For this review, take the finished solid that the model builds, in its own axes (mm). A direction names the side the tool comes from. Round coordinates to 2 decimals unless told otherwise and drop trailing zeros. Order: outer loops, then holes, each group sorted by start corner. A loop starts at its lowest first (then second) coordinate and runs counter-clockwise, first axis right, second up. Notation, with made-up numbers: (41.5, 81.25) -> (71.5, 81.25) arc R24 ccw to (71.5, 101.25) -> close; hole circle Ø9 at (-36, 10). An arc over 180 degrees is marked (long way). Use a Markdown table: item, result. Add a question column.
1) Wall thickness on line 1 along Y through (x, z) = (-21, 17); line 2 along X through (y, z) = (-2, 20.25); line 3 along Y through (x, z) = (-56, 3.5): over which ranges is each line inside the solid? List them lowest first. Write a range as [from, to].
2) Clearance check with flat-ended pins moving along their axes: P1, Ø2, axis at x = -53.6, z = 9.38, coming from the +Y side; P2, Ø5, axis at y = -20.5, z = 8.5, coming from the -X side; P3, Ø3, axis at y = -3.5, z = 14, coming from the +X side; P4, Ø4, axis at x = -54, z = 10.5, coming from the -Y side. State where each tip first meets the part, or that it passes through.
3) Machinability: for faces 4 (the face through (-10.201, -4, 18)), 5 (the face through (-55.077, -7.64, 8.434)), 6 (the face through (-54, -6.119, 14)), 7 (the face through (-28.201, -4, 15)), 8 (the face through (-54, -9.119, 14)), which of the approach directions +Z, -Z, +X, -X, +Y, -Y give a long, thin tool a straight path to every point of the face, cutting with its end or side? Answer none if there is none.
4) Consider section A-A (z = 19.5). State the section outline as (x, y) points, plus the area to 3 significant figures.
5) Consider section C-C (y = 2). State the section outline as (x, z) points, plus the area to 3 significant figures.
6) Draft analysis for pull direction Y (two halves, no side actions). For faces 1 (the face through (-21.87, -4.46, 5.98)), 2 (the face through (-50.401, 6, 14)), 3 (the face through (-31, 17.781, 14)), state which applies: pulls with the +Y half, pulls with the -Y half, needs draft (parallel to the pull), parting line crosses it, or undercut.
7) Consider section D-D (z = 5). State the section outline as (x, y) points.
8) Consider section B-B (x = -40.5). State the section outline as (y, z) points, plus the area to 3 significant figures.
```python
from build123d import *

# Parameters (mm, degrees)
SKETCH2_W               = 40.2
SKETCH2_H               = 43.15
BOSS_EXTRUDE1_DEPTH     = 29.13
SKETCH3_W               = 29.13
SKETCH3_H               = 3
BOSS_EXTRUDE2_DEPTH     = 8
CUT_EXTRUDE1_DEPTH      = 8
CUT_EXTRUDE1_DEPTH_BACK = 8
SKETCH4_R               = 1.75
SKETCH5_R               = 1.75
CUT_EXTRUDE2_DEPTH      = 40
SKETCH6_R               = 3
CUT_EXTRUDE3_DEPTH      = 18


with BuildPart() as part:
    # Sketch2 → Boss-Extrude1 (new body)
    with BuildSketch(Plane.XY):
        with Locations((-30.301325873, -3.793821583)):
            Rectangle(SKETCH2_W, SKETCH2_H)
    extrude(amount=BOSS_EXTRUDE1_DEPTH)

    # Sketch3 → Boss-Extrude2 (add)
    with BuildSketch(Plane.ZY.offset(50.401325873)):
        with Locations((14.565, -7.618821583)):
            Rectangle(SKETCH3_W, SKETCH3_H)
    extrude(amount=BOSS_EXTRUDE2_DEPTH)

    # Sketch4 → Cut-Extrude1 (cut, two sides: drawn at the far end of the back side and taken through both)
    with BuildSketch(Plane(origin=(0, -9.118821583, 0), x_dir=(1, 0, 0), z_dir=(0, 1, 0)).offset(-CUT_EXTRUDE1_DEPTH_BACK)):
        with Locations(Location((-53.601325886, -9.375, 0), (0, 0, 90))):
            Circle(SKETCH4_R)
        with Locations(Location((-53.601325886, -19.725, 0), (0, 0, 90))):
            Circle(SKETCH4_R)
    extrude(amount=CUT_EXTRUDE1_DEPTH + CUT_EXTRUDE1_DEPTH_BACK, mode=Mode.SUBTRACT)

    # Sketch5 → Cut-Extrude2 (cut)
    with BuildSketch(Plane(origin=(0, 0, 0), x_dir=(-1, 0, 0), z_dir=(0, 0, -1))):
        with Locations((40.351325873, -3.793821583)):
            Circle(SKETCH5_R)
        with Locations((20.251325873, -3.793821583)):
            Circle(SKETCH5_R)
    extrude(amount=-CUT_EXTRUDE2_DEPTH, mode=Mode.SUBTRACT)

    # Sketch6 → Cut-Extrude3 (cut)
    with BuildSketch(Plane(origin=(-10.201325873, 0, 0), x_dir=(0, 0, -1), z_dir=(1, 0, 0))):
        with Locations((-14.565, -3.793821583)):
            Circle(SKETCH6_R)
    extrude(amount=-CUT_EXTRUDE3_DEPTH, mode=Mode.SUBTRACT)


solid = part.part
```
Results list:
| question | item | result |
|---|---|---|
| 1 | line 1 | [-25.37, -5.55], [-2.04, 17.78] |
| 1 | line 2 | [-50.4, -10.2] |
| 1 | line 3 | [-9.12, -6.12] |
| 2 | P1 | through |
| 2 | P2 | x = -50.4 |
| 2 | P3 | x = -28.2 |
| 2 | P4 | y = -9.12 |
| 3 | face 4 | +Z, -Z, +X, +Y, -Y |
| 3 | face 5 | +Y, -Y |
| 3 | face 6 | +Z, -Z, -X, +Y |
| 3 | face 7 | +X |
| 3 | face 8 | +Z, -Z, -X, -Y |
| 4 | outline | (-58.4, -9.12) -> (-55.34, -9.12) -> (-55.34, -6.12) -> (-58.4, -6.12) -> close; (-51.87, -9.12) -> (-50.4, -9.12) -> (-50.4, -25.37) -> (-10.2, -25.37) -> (-10.2, 17.78) -> (-50.4, 17.78) -> (-50.4, -6.12) -> (-51.87, -6.12) -> close; hole circle Ø3.5 at (-40.35, -3.79); hole circle Ø3.5 at (-20.25, -3.79) |
| 4 | area | 1,730 mm2 |
| 5 | outline | (-50.4, 0) -> (-10.2, 0) -> (-10.2, 29.13) -> (-50.4, 29.13) -> close |
| 5 | area | 1,170 mm2 |
| 6 | face 1 | undercut |
| 6 | face 2 | needs draft |
| 6 | face 3 | pulls with the +Y half |
| 7 | outline | (-58.4, -9.12) -> (-50.4, -9.12) -> (-50.4, -25.37) -> (-10.2, -25.37) -> (-10.2, 17.78) -> (-50.4, 17.78) -> (-50.4, -6.12) -> (-58.4, -6.12) -> close; hole circle Ø3.5 at (-40.35, -3.79); hole circle Ø3.5 at (-20.25, -3.79) |
| 8 | outline | (-25.37, 0) -> (-5.54, 0) -> (-5.54, 29.13) -> (-25.37, 29.13) -> close; (-2.05, 0) -> (17.78, 0) -> (17.78, 29.13) -> (-2.05, 29.13) -> close |
| 8 | area | 1,160 mm2 |
